```python
from build123d import *

# Parameters (mm, degrees)
F0_R     = 10.9982
F1_DEPTH = 7.62


with BuildPart() as f1:
    # F0 (on Front) → F1 (new body)
    with BuildSketch(Plane.XZ):
        with BuildLine():
            ThreePointArc((-10.9982, 0), (-7.7769018008, 7.7769018008), (0, 10.9982))
            Line((0, 10.9982), (0, 17.78))
            ThreePointArc((0, 17.78), (-5.3788561382, 18.7607746829), (-10.0653965385, 21.5768626451))
            ThreePointArc((-10.0653965385, 21.5768626451), (-11.9253757257, 17.0869306915), (-16.4153965312, 15.2271660045))
            Line((-16.4153965312, 15.2271660045), (-32.3946877004, 15.2271660045))
            ThreePointArc((-32.3946877004, 15.2271660045), (-22.0248338019, 10.5529105121), (-17.78, 0))
            Line((-17.78, 0), (-10.9982, 0))
        make_face()
        with BuildLine():
            Line((0, 17.78), (0, 10.9982))
            ThreePointArc((0, 10.9982), (7.7769018008, 7.7769018008), (10.9982, 0))
            Line((10.9982, 0), (17.78, 0))
            ThreePointArc((17.78, 0), (23.4843953598, 11.8882229179), (36.3272236413, 14.8768233097))
            Line((36.3272236413, 14.8768233097), (20.2106650558, 18.459648921))
            ThreePointArc((20.2106650558, 18.459648921), (16.6352486905, 20.6851567), (15.2386749063, 24.6583253))
            Line((15.2386749063, 24.6583253), (15.2386749063, 32.8190345816))
            ThreePointArc((15.2386749063, 32.8190345816), (10.7050195475, 22.1728733534), (0, 17.78))
        make_face()
        with BuildLine():
            ThreePointArc((0, -10.9982), (-7.7769018008, -7.7769018008), (-10.9982, 0))
            Line((-10.9982, 0), (-17.78, 0))
            ThreePointArc((-17.78, 0), (-22.2436926547, -10.7763073453), (-33.02, -15.24))
            Line((-33.02, -15.24), (-21.59, -15.24))
            ThreePointArc((-21.59, -15.24), (-17.0998719395, -17.0998719395), (-15.24, -21.59))
            Line((-15.24, -21.59), (-15.24, -33.02))
            ThreePointArc((-15.24, -33.02), (-10.7763073453, -22.2436926547), (0, -17.78))
            Line((0, -17.78), (0, -10.9982))
        make_face()
        with BuildLine():
            Line((17.78, 0), (10.9982, 0))
            ThreePointArc((10.9982, 0), (7.7769018008, -7.7769018008), (0, -10.9982))
            Line((0, -10.9982), (0, -17.78))
            ThreePointArc((0, -17.78), (10.7763073453, -22.2436926547), (15.24, -33.02))
            Line((15.24, -33.02), (15.24, -21.59))
            ThreePointArc((15.24, -21.59), (17.0998719395, -17.0998719395), (21.59, -15.24))
            Line((21.59, -15.24), (33.02, -15.24))
            ThreePointArc((33.02, -15.24), (22.2436926547, -10.7763073453), (17.78, 0))
        make_face()
        with BuildLine():
            ThreePointArc((-10.0653965385, 21.5768626451), (-5.3788561382, 18.7607746829), (0, 17.78))
            Line((0, 17.78), (0, 22.0218))
            ThreePointArc((0, 22.0218), (-7.5754508533, 25.0467354485), (-10.9838107601, 32.4575905169))
            Line((-10.9838107601, 32.4575905169), (-10.9838107601, 24.8666))
            ThreePointArc((-10.9838107601, 24.8666), (-10.2992675476, 23.2846396517), (-10.0653965385, 21.5768626451))
        make_face()
        with BuildLine():
            Line((0, 22.0218), (0, 17.78))
            ThreePointArc((0, 17.78), (10.7050195475, 22.1728733534), (15.2386749063, 32.8190345816))
            ThreePointArc((15.2386749063, 32.8190345816), (15.239668723, 32.9195151065), (15.24, 33.02))
            ThreePointArc((15.24, 33.02), (14.6261956768, 37.301588493), (12.8342257188, 41.2382875467))
            ThreePointArc((12.8342257188, 41.2382875467), (0, 48.26), (-12.8342257188, 41.2382875467))
            ThreePointArc((-12.8342257188, 41.2382875467), (-15.091092809, 30.894789933), (-10.0653965385, 21.5768626451))
            ThreePointArc((-10.0653965385, 21.5768626451), (-10.2992675476, 23.2846396517), (-10.9838107601, 24.8666))
            Line((-10.9838107601, 24.8666), (-10.9838107601, 32.4575905169))
            ThreePointArc((-10.9838107601, 32.4575905169), (-0.2812967636, 44.0146021015), (10.9982, 33.02))
            ThreePointArc((10.9982, 33.02), (7.7769018008, 25.2430981992), (0, 22.0218))
        make_face()
        with BuildLine():
            ThreePointArc((-33.02, -15.24), (-22.2436926547, -10.7763073453), (-17.78, 0))
            ThreePointArc((-17.78, 0), (-22.0248338019, 10.5529105121), (-32.3946877004, 15.2271660045))
            Line((-32.3946877004, 15.2271660045), (-33.6453122996, 15.2271660045))
            ThreePointArc((-33.6453122996, 15.2271660045), (-38.2946425734, 14.2981028714), (-42.4334579703, 11.985174552))
            ThreePointArc((-42.4334579703, 11.985174552), (-48.26, 0), (-42.4334579703, -11.985174552))
            ThreePointArc((-42.4334579703, -11.985174552), (-38.0001375397, -14.4033270492), (-33.02, -15.24))
        make_face()
        with Locations((-33.02, 0)):
            Circle(F0_R, mode=Mode.SUBTRACT)
        with BuildLine():
            ThreePointArc((36.3272236413, 14.8768233097), (23.4843953598, 11.8882229179), (17.78, 0))
            ThreePointArc((17.78, 0), (22.2436926547, -10.7763073453), (33.02, -15.24))
            ThreePointArc((33.02, -15.24), (37.6384409366, -14.5233468359), (41.8225222525, -12.4407878366))
            ThreePointArc((41.8225222525, -12.4407878366), (46.555287938, -7.0038261283), (48.26, 0))
            ThreePointArc((48.26, 0), (46.5542268134, 7.0058764309), (41.8187526818, 12.4434541525))
            ThreePointArc((41.8187526818, 12.4434541525), (39.1940575837, 13.9333633037), (36.3272236413, 14.8768233097))
        make_face()
        with BuildLine():
            ThreePointArc((44.0182, 0), (33.02, -10.9982), (22.0218, 0))
            ThreePointArc((22.0218, 0), (33.02, 10.9982), (44.0182, 0))
        make_face(mode=Mode.SUBTRACT)
        with BuildLine():
            ThreePointArc((15.24, -33.02), (10.7763073453, -22.2436926547), (0, -17.78))
            ThreePointArc((0, -17.78), (-10.7763073453, -22.2436926547), (-15.24, -33.02))
            ThreePointArc((-15.24, -33.02), (-14.730806545, -36.9265251226), (-13.2372521609, -40.5720033917))
            Line((-13.2372521609, -40.5720033917), (-12.0341089163, -42.370819354))
            ThreePointArc((-12.0341089163, -42.370819354), (0, -48.26), (12.0341089163, -42.370819354))
            Line((12.0341089163, -42.370819354), (13.2372521609, -40.5720033917))
            ThreePointArc((13.2372521609, -40.5720033917), (14.730806545, -36.9265251226), (15.24, -33.02))
        make_face()
        with BuildLine():
            ThreePointArc((10.9982, -33.02), (-7.7769018008, -40.7969018008), (0, -22.0218))
            ThreePointArc((0, -22.0218), (7.7769018008, -25.2430981992), (10.9982, -33.02))
        make_face(mode=Mode.SUBTRACT)
        with BuildLine():
            Line((-33.6453122996, 15.2271660045), (-32.3946877004, 15.2271660045))
            ThreePointArc((-32.3946877004, 15.2271660045), (-33.02, 15.24), (-33.6453122996, 15.2271660045))
        make_face()
        with BuildLine():
            Line((0, 61.2810700441), (-12.8342257188, 41.2382875467))
            ThreePointArc((-12.8342257188, 41.2382875467), (0, 48.26), (12.8342257188, 41.2382875467))
            Line((12.8342257188, 41.2382875467), (0, 61.2810700441))
        make_face()
        with BuildLine():
            Line((-63.0083821844, 0), (-42.4334579703, -11.985174552))
            ThreePointArc((-42.4334579703, -11.985174552), (-48.26, 0), (-42.4334579703, 11.985174552))
            Line((-42.4334579703, 11.985174552), (-63.0083821844, 0))
        make_face()
        with BuildLine():
            Line((62.1118612768, 0), (41.8187526818, 12.4434541525))
            ThreePointArc((41.8187526818, 12.4434541525), (46.5542268134, 7.0058764309), (48.26, 0))
            ThreePointArc((48.26, 0), (46.555287938, -7.0038261283), (41.8225222525, -12.4407878366))
            Line((41.8225222525, -12.4407878366), (62.1118612768, 0))
        make_face()
        with BuildLine():
            ThreePointArc((12.0341089163, -42.370819354), (12.6676500342, -41.4927942622), (13.2372521609, -40.5720033917))
            Line((13.2372521609, -40.5720033917), (12.0341089163, -42.370819354))
        make_face()
        with BuildLine():
            Line((-12.0341089163, -42.370819354), (-13.2372521609, -40.5720033917))
            ThreePointArc((-13.2372521609, -40.5720033917), (-12.6676500342, -41.4927942622), (-12.0341089163, -42.370819354))
        make_face()
        with BuildLine():
            Line((0, -60.3629805593), (12.0341089163, -42.370819354))
            ThreePointArc((12.0341089163, -42.370819354), (0, -48.26), (-12.0341089163, -42.370819354))
            Line((-12.0341089163, -42.370819354), (0, -60.3629805593))
        make_face()
    extrude(amount=F1_DEPTH)


solid = f1.part
```
Geometry check sheet. Reference: the model listing, model coordinates, mm. A direction names the side the tool comes from. Give positions to 0.01 mm unless a question says otherwise; leave off trailing zeros. Write each loop counter-clockwise with the first axis right and the second up, starting at its lowest first coordinate (ties: lowest second). Pieces come first, ordered by that corner, then holes.
1) Section check B-B, the plane z = -23.5. Record the boundary of the cut face in (x, y), and give its area (3 significant figures).
2) Material ranges on L1, parallel to Z at x = -33.02, y = -6; L2, parallel to Z at x = -8, y = -1.25, recorded low to high.
3) Gauge pin test, flat ends, axial feed: pin 1 (4 mm diameter, centred on x = -25.5, y = -4.5, fed in from -Z); pin 2 (2.5 mm diameter, centred on y = -3, z = 27, fed in from +X); pin 3 (2 mm diameter, centred on y = -3, z = 42, fed in from -X). Record the tip position at first contact, or that the pin passes through.
4) Section check D-D, the plane z = 47. Record the boundary of the cut face in (x, y).
5) Access from +Z, -Z, +X, -X, +Y, -Y to the whole of each face (thin tool, end or side, straight path). Record for faces 1 (the flat face through (15.24, -4, -27)), 2 (the flat face through (15.239, -4, 29)), 3 (the flat face through (-27, -4, -15.24)), 4 (the flat face through (-24, -4, 15.227)).
6) Section check A-A, the plane x = 9.5. Record the boundary of the cut face in (y, z).
7) Section check C-C, the plane y = -1.5. State how many separate pieces and enclosed holes the cut face has, and give its area (3 significant figures).
Computed:
1. outline: (-15.24, -7.62) - (-5.51, -7.62) - (-5.51, 0) - (-15.24, 0) - close; (5.51, -7.62) - (15.24, -7.62) - (15.24, 0) - (5.51, 0) - close
1. area: 148 mm2
2. L1: z = -15.24 to -11, 11 to 15.24
2. L2: z = -48.4 to -40.57, -25.47 to -7.55, 7.55 to 25.47, 40.57 to 48.79
3. pin 1: stops at z = -15.24
3. pin 2: stops at x = 15.24
3. pin 3: stops at x = -12.98
4. outline: (-9.14, -7.62) - (9.14, -7.62) - (9.14, 0) - (-9.14, 0) - close
5. face 1: -Z, +X, +Y, -Y
5. face 2: +Z, +X, +Y, -Y
5. face 3: -Z, -X, +Y, -Y
5. face 4: +Z, -X, +Y, -Y
6. outline: (-7.62, -46.16) - (0, -46.16) - (0, -38.56) - (-7.62, -38.56) - close; (-7.62, -27.48) - (0, -27.48) - (0, -5.54) - (-7.62, -5.54) - close; (-7.62, 5.54) - (0, 5.54) - (0, 27.48) - (-7.62, 27.48) - close; (-7.62, 38.56) - (0, 38.56) - (0, 46.45) - (-7.62, 46.45) - close
7. separate pieces: 1
7. enclosed holes: 5
7. area: 3,220 mm2
